Autodesk Inventor part; units mm, degrees
ref_plane "YZ Plane" through (0, 0, 0) normal (1, 0, 0) x (0, 1, 0)
ref_plane "XZ Plane" through (0, 0, 0) normal (0, 1, 0) x (-1, 0, 0)
ref_plane "XY Plane" through (0, 0, 0) normal (0, 0, 1) x (1, 0, 0)
sketch "Sketch1" plane through (0, 0, 0) normal (1, 0, 0) x (0, 1, 0)
  circle A0 centre (0, 0) radius 4
  dimension "d0" = 4
extrude "Extrusion1" add sketch "Sketch1" along normal blind 150
sketch "Sketch2" plane through (150, 0, 0) normal (1, 0, 0) x (0, 0, -1)
  circle A0 centre (0, 0) radius 4
  line L0 (0, 7.5056) -> (6.5, 3.7528)
  line L1 (6.5, 3.7528) -> (6.5, -3.7528)
  line L2 (6.5, -3.7528) -> (0, -7.5056)
  line L3 (0, -7.5056) -> (-6.5, -3.7528)
  line L4 (-6.5, -3.7528) -> (-6.5, 3.7528)
  line L5 (-6.5, 3.7528) -> (0, 7.5056)
  dimension "d5" = 13
  dimension "d8" = 6.5
thread "Thread2"
extrude "Extrusion2" add sketch "Sketch2" along normal blind 5 contours A0 | L0 L1 L2 L3 L4 L5
chamfer "Chamfer1" distance 1 angle 45 1 edges at (0, -4, 0)
properties part number "M8x150mm"
Input: part model. Units: mm. Frame: model coordinates. A direction names the side the tool comes from. Coordinates: 2 decimals unless noted, no trailing zeros. Order: outer loops, then holes, each group sorted by start corner. A loop starts at its lowest first (then second) coordinate and runs counter-clockwise, first axis right, second up. Notation, with made-up numbers: M -20,-34.75 L 20,-34.75 A10 ccw 20,-16.75 Z; hole C 72,71.5 d10. An arc over 180 degrees is marked long. Write item = value, one per line. Start each with the question number.
(1) Line query: line 1 along X through (y, z) = (0.5, 5.5); line 2 along Z through (x, y) = (118, -0.5); line 3 along Y through (x, z) = (17, 3). Output: solid intervals per line, ascending. Write a range as [from, to].
(2) Section A-A on y = 0. Output: boundary loops of the cut face in (x, z), and give its area (3 significant figures).
(3) Reachability of faces 1 (the cylindrical face through (74.457, -0.867, 3.905)), 2 (the flat face through (152.5, -5.6, -3.3)) from +Z, -Z, +X, -X, +Y, -Y: full face, straight path, thin tool, end or side. Return the list, or none.
(4) Section B-B on x = 58. Output: boundary loops of the cut face in (y, z).
(5) First-contact query: P1, Ø6, axis at x = 95.5, y = 0.5, coming from the +Z side; P2, Ø1, axis at x = 23, y = -0.5, coming from the -Z side; P3, Ø4, axis at y = 1.5, z = 0.5, coming from the -X side. Flat tips, straight axial feed; report the tip coordinate or a pass-through.
Result set:
q1.line_1 = [150, 155]
q1.line_2 = [-3.97, 3.97]
q1.line_3 = [-2.65, 2.65]
q2.outline = M 0,-3 L 1,-4 L 150,-4 L 150,-6.5 L 155,-6.5 L 155,6.5 L 150,6.5 L 150,4 L 1,4 L 0,3 Z
q2.area = 1,260 mm²
q3.face_1 = -X
q3.face_2 = -Z, +X, -X, -Y
q4.outline = C 0,0 d8
q5.P1 = 4
q5.P2 = -4
q5.P3 = 0
